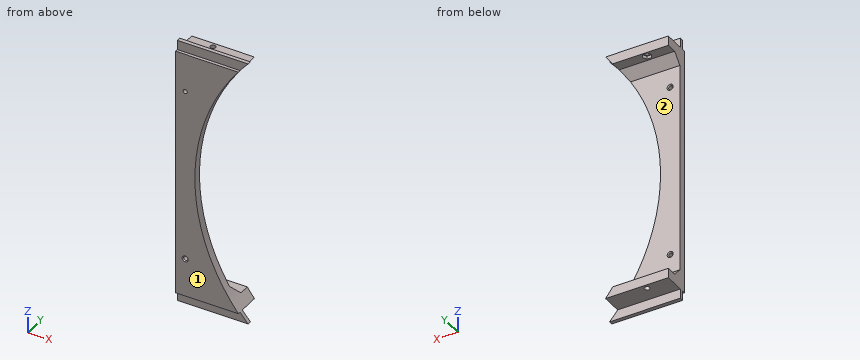
from build123d import *

# Parameters (mm, degrees)
SKETCH1_W                = 650
SKETCH1_H                = 650
BOSS_EXTRUDE1_DEPTH      = 8
BOSS_EXTRUDE2_DEPTH      = 650
CUT_EXTRUDE2_DEPTH       = 921.277302922
CUT_EXTRUDE2_DEPTH_BACK  = 921.277302922
SKETCH4_R                = 11
CUT_EXTRUDE1_DEPTH       = 920.932062709
CUT_EXTRUDE1_DEPTH_BACK  = 920.932062709
SKETCH2_R                = 210
CUT_EXTRUDE3_DEPTH       = 921.277302998
CUT_EXTRUDE3_DEPTH_BACK  = 110
CUT_EXTRUDE4_DEPTH       = 110
CUT_EXTRUDE5_DEPTH       = 920.932062713
CUT_EXTRUDE5_DEPTH_BACK  = 920.932062713
SKETCH7_OUTSIDE_W        = 836.056
SKETCH7_OUTSIDE_H        = 836.056
BOSS_EXTRUDE3_DEPTH      = 170
SKETCH11_W               = 9.9
SKETCH11_H               = 4
BOSS_EXTRUDE4_DEPTH      = 170
CUT_EXTRUDE7_DEPTH       = 496.410950626
CUT_EXTRUDE7_DEPTH_BACK  = 496.410950626
SKETCH10_R               = 210
CUT_EXTRUDE8_DEPTH       = 320.349035711
CUT_EXTRUDE8_DEPTH_BACK  = 320.349035711
SKETCH12_R               = 2.75
SKETCH12_R_2             = 2.2
CUT_EXTRUDE9_DEPTH       = 495.859380642
CUT_EXTRUDE9_DEPTH_BACK  = 495.859380642
SKETCH13_W               = 95
SKETCH13_H               = 279.8
CUT_EXTRUDE10_DEPTH      = 495.859380642
CUT_EXTRUDE10_DEPTH_BACK = 495.859380642
SKETCH14_R               = 2.15
CHAMFER1_SIZE            = 1
CUT_EXTRUDE11_DEPTH      = 3
LPATTERN1_COUNT          = 2
LPATTERN1_PITCH          = 243


with BuildPart() as part:
    # Sketch1 → Boss-Extrude1 (new body)
    with BuildSketch(Plane(origin=(0, 0, 0), x_dir=(1, 0, 0), z_dir=(0, 1, 0))):
        with Locations((325, 325)):
            Rectangle(SKETCH1_W, SKETCH1_H)
    extrude(amount=BOSS_EXTRUDE1_DEPTH)

    # Sketch3 → Boss-Extrude2 (add)
    with BuildSketch(Plane.XY):
        Polygon((300, 43.707142143), (350, 43.707142143), (385, 8), (265, 8), align=None)
    extrude(amount=-BOSS_EXTRUDE2_DEPTH)

    # Sketch4 → Cut-Extrude2 (cut, two sides: drawn at the far end of the back side and taken through both)
    with BuildSketch(Plane.XY.offset(-CUT_EXTRUDE2_DEPTH_BACK)):
        with Locations((325, 22)):
            Circle(SKETCH4_R)
    extrude(amount=CUT_EXTRUDE2_DEPTH + CUT_EXTRUDE2_DEPTH_BACK, mode=Mode.SUBTRACT)

    # Sketch2 → Cut-Extrude1 (cut, two sides: drawn at the far end of the back side and taken through both)
    with BuildSketch(Plane(origin=(0, 8, 0), x_dir=(1, 0, 0), z_dir=(0, 1, 0)).offset(-CUT_EXTRUDE1_DEPTH_BACK)):
        with Locations(Location((325, 325, 0), (0, 0, 270))):
            Circle(SKETCH2_R)
    extrude(amount=CUT_EXTRUDE1_DEPTH + CUT_EXTRUDE1_DEPTH_BACK, mode=Mode.SUBTRACT)

    # Sketch5 → Cut-Extrude3 (cut, two sides: drawn at the far end of the back side and taken through both)
    with BuildSketch(Plane.XY.offset(-CUT_EXTRUDE3_DEPTH_BACK)):
        Polygon((300, 43.707142143), (350, 43.707142143), (365.396078824, 28), (350, 28), (350, 8), (300, 8), (300, 28), (284.603921176, 28), align=None)
    extrude(amount=CUT_EXTRUDE3_DEPTH + CUT_EXTRUDE3_DEPTH_BACK, mode=Mode.SUBTRACT)

    # Sketch6 → Cut-Extrude4 (cut)
    with BuildSketch(Plane(origin=(0, 0, -650), x_dir=(-1, 0, 0), z_dir=(0, 0, -1))):
        Polygon((-350, 43.707142143), (-300, 43.707142143), (-284.603921176, 28), (-300, 28), (-300, 8), (-350, 8), (-350, 28), (-365.396078824, 28), align=None)
    extrude(amount=-CUT_EXTRUDE4_DEPTH, mode=Mode.SUBTRACT)

    # Sketch7 outside → Cut-Extrude5 (cut, two sides: drawn at the far end of the back side and taken through both)
    with BuildSketch(Plane(origin=(0, 8, 0), x_dir=(1, 0, 0), z_dir=(0, 1, 0)).offset(-CUT_EXTRUDE5_DEPTH_BACK)):
        with Locations((325, 325)):
            Rectangle(SKETCH7_OUTSIDE_W, SKETCH7_OUTSIDE_H)
        Polygon((195, 455), (-124.314954955, 455), (-40.613333333, 195), (195, 195), align=None, mode=Mode.SUBTRACT)
    extrude(amount=CUT_EXTRUDE5_DEPTH + CUT_EXTRUDE5_DEPTH_BACK, mode=Mode.SUBTRACT)

    # Sketch8 → Boss-Extrude3 (add)
    with BuildSketch(Plane.ZY):
        Polygon((-455, 8), (-455, 28), (-445, 28), (-445, 17), (-435, 8), align=None)
        Polygon((-195, 8), (-195, 28), (-205, 28), (-205, 17), (-215, 8), align=None)
    extrude(amount=-BOSS_EXTRUDE3_DEPTH)

    # Sketch11 → Boss-Extrude4 (add)
    with BuildSketch(Plane.ZY):
        with Locations((-459.95, 5)):
            Rectangle(SKETCH11_W, SKETCH11_H)
        with Locations((-190.05, 5)):
            Rectangle(SKETCH11_W, SKETCH11_H)
    extrude(amount=-BOSS_EXTRUDE4_DEPTH)

    # Sketch10 → Cut-Extrude7 (cut, two sides: drawn at the far end of the back side and taken through both)
    with BuildSketch(Plane(origin=(0, 8, 0), x_dir=(1, 0, 0), z_dir=(0, 1, 0)).offset(-CUT_EXTRUDE7_DEPTH_BACK)):
        with Locations((325, 325)):
            Circle(SKETCH10_R)
    extrude(amount=CUT_EXTRUDE7_DEPTH + CUT_EXTRUDE7_DEPTH_BACK, mode=Mode.SUBTRACT)

    # Sketch12 → Cut-Extrude8 (cut, two sides: drawn at the far end of the back side and taken through both)
    with BuildSketch(Plane.XY.offset(-195).offset(-CUT_EXTRUDE8_DEPTH_BACK)):
        with Locations((40, 23)):
            Circle(SKETCH12_R)
        with Locations((80, 23)):
            Circle(SKETCH12_R_2)
        with Locations((120, 23)):
            Circle(SKETCH12_R)
    extrude(amount=CUT_EXTRUDE8_DEPTH + CUT_EXTRUDE8_DEPTH_BACK, mode=Mode.SUBTRACT)

    # Sketch13 → Cut-Extrude9 (cut, two sides: drawn at the far end of the back side and taken through both)
    with BuildSketch(Plane(origin=(0, 8, 0), x_dir=(1, 0, 0), z_dir=(0, 1, 0)).offset(-CUT_EXTRUDE9_DEPTH_BACK)):
        with Locations((47.5, 325)):
            Rectangle(SKETCH13_W, SKETCH13_H)
    extrude(amount=CUT_EXTRUDE9_DEPTH + CUT_EXTRUDE9_DEPTH_BACK, mode=Mode.SUBTRACT)

    # Sketch14 → Cut-Extrude10 (cut, two sides: drawn at the far end of the back side and taken through both)
    with BuildSketch(Plane(origin=(0, 8, 0), x_dir=(1, 0, 0), z_dir=(0, 1, 0)).offset(-CUT_EXTRUDE10_DEPTH_BACK)):
        with Locations(Location((105, 235, 0), (0, 0, 270))):
            Circle(SKETCH14_R)
        with Locations(Location((105, 415, 0), (0, 0, 270))):
            Circle(SKETCH14_R)
    extrude(amount=CUT_EXTRUDE10_DEPTH + CUT_EXTRUDE10_DEPTH_BACK, mode=Mode.SUBTRACT)

    # Chamfer1
    chamfer1_edges = [part.edges().sort_by_distance(p)[0] for p in [
        (105, 8, -237.15),
        (105, 0, -417.15),
        (105, 8, -417.15),
    ]]
    chamfer(chamfer1_edges, length=CHAMFER1_SIZE)

    # Sketch15 → Cut-Extrude11 (cut)
    with BuildSketch(Plane(origin=(0, 0, -205), x_dir=(-1, 0, 0), z_dir=(0, 0, -1))):
        Polygon((-122.367136104, 27.1), (-117.632863896, 27.1), (-115.265727793, 23), (-117.632863896, 18.9), (-122.367136104, 18.9), (-124.734272207, 23), align=None)
    cut_extrude11 = extrude(amount=-CUT_EXTRUDE11_DEPTH, mode=Mode.SUBTRACT)

    # LPattern1: Cut-Extrude11 ×2
    with Locations(*[(0, 0, -i * LPATTERN1_PITCH) for i in range(1, LPATTERN1_COUNT)]):
        add(cut_extrude11, mode=Mode.SUBTRACT)


solid = part.part
Here's how the part is built. I have some questions about the finished solid (model axes, mm). Face numbers are marked on the shaded views. Give positions to 0.01 mm unless a question says otherwise; leave off trailing zeros. Order: outer loops, then holes, each group sorted by start corner. A loop starts at its lowest first (then second) coordinate and runs counter-clockwise, first axis right, second up. Notation, with made-up numbers: (60, 24.25) -> (66, 24.25) arc R12 cw to (66, 30.25) -> close; hole circle Ø1 at (43.25, 58). An arc over 180 degrees is marked (long way). Use a Markdown table: item, result. Add a question column.
Item 1: Imagine slicing it at C-C on z = -358. Please give me the cut outline in (x, y).
Item 2: Imagine slicing it at D-D on z = -273.5. Please give me the cut outline in (x, y), plus the area to 3 significant figures.
Item 3: Imagine slicing it at A-A on x = 134. Please give me the cut outline in (y, z).
Item 4: If we mould it in two halves opening along Z, with no side actions, what happens to the marked faces 1 and 2? For each: pulls with the +Z half, pulls with the -Z half, needs draft (parallel to the pull), parting line crosses it, or undercut.
Item 5: Imagine slicing it at B-B on x = 120. Give the number of separate pieces and of enclosed holes in the cut face, plus the area to 3 significant figures.
Item 6: Will these pins go through, and if not, where does the flat tip stop? pin 1 (8 mm diameter, centred on x = 154, y = 14.5, fed in from +Z); pin 2 (10.5 mm diameter, centred on x = 125.5, y = 21.5, fed in from -Z); pin 3 (2 mm diameter, centred on x = 120.5, z = -429.5, fed in from -Y); pin 4 (5 mm diameter, centred on x = 130, z = -459.5, fed in from +Y).
Item 7: I need wall thicknesses on line 1 (Z direction, x = 105, y = 5.05); line 2 (Z direction, x = 105, y = 2.85); line 3 (Z direction, x = 114.5, y = 20.5). Which ranges of each line are inside material? Lowest first, please.
Data:
| question | item | result |
|---|---|---|
| 1 | outline | (95, 0) -> (117.61, 0) -> (117.61, 8) -> (95, 8) -> close |
| 2 | outline | (95, 0) -> (121.41, 0) -> (121.41, 8) -> (95, 8) -> close |
| 2 | area | 211 mm² |
| 3 | outline | (0, -455) -> (3, -455) -> (3, -464.9) -> (7, -464.9) -> (7, -455) -> (28, -455) -> (28, -445) -> (17, -445) -> (8, -435) -> (8, -412.29) -> (0, -412.29) -> close; (0, -237.71) -> (8, -237.71) -> (8, -215) -> (17, -205) -> (28, -205) -> (28, -195) -> (7, -195) -> (7, -185.1) -> (3, -185.1) -> (3, -195) -> (0, -195) -> close |
| 4 | face 1 | needs draft |
| 4 | face 2 | undercut |
| 5 | separate pieces | 4 |
| 5 | enclosed holes | 0 |
| 5 | area | 1,790 mm² |
| 6 | pin 1 | stops at z = -195 |
| 6 | pin 2 | stops at z = -455 |
| 6 | pin 3 | stops at y = 0 |
| 6 | pin 4 | stops at y = 7 |
| 7 | line 1 | z = -464.9 to -417.15, -412.85 to -237.15, -232.85 to -185.1 |
| 7 | line 2 | z = -455 to -417.15, -412.85 to -237.15, -232.85 to -195 |
| 7 | line 3 | z = -455 to -445, -205 to -195 |
